Check sheet for the modelled part. Datum: model origin and axes. Units: mm. Face numbers are marked on the shaded views. Give positions to 0.01 mm unless a question says otherwise; leave off trailing zeros. Order: outer loops, then holes, each group sorted by start corner. A loop starts at its lowest first (then second) coordinate and runs counter-clockwise, first axis right, second up.
Item 1: Gauge pin test, flat ends, axial feed: P1, Ø5, axis at y = -15.5, z = 6.5, coming from the +X side; P2, Ø10, axis at x = 28.5, y = -17, coming from the +Z side; P3, Ø3, axis at y = -9.5, z = -18.5, coming from the +X side; P4, Ø6, axis at y = -6, z = -3, coming from the -X side. Record the tip position at first contact, or that the pin passes through.
Item 2: Release check for a two-part mould opening along X. For the marked faces 1 and 2 record: released by +X, released by -X, zero draft, split by the parting line, or undercut.
Item 3: Sectioned sample at A-A on z = -19. Record the boundary of the cut face in (x, y), and give its area (3 significant figures).
Item 4: Material ranges on line 1 along X through (y, z) = (-4, -26.5); line 2 along X through (y, z) = (-16.5, 43); line 3 along Z through (x, y) = (36, -18), recorded low to high.
Item 5: Sectioned sample at C-C on y = -18.25. Record the boundary of the cut face in (x, z), and give its area (3 significant figures).
Item 6: Sectioned sample at B-B on x = -20.5. Record the boundary of the cut face in (y, z), and give its area (3 significant figures).
Item 7: Sectioned sample at D-D on z = 0. Record the boundary of the cut face in (x, y), and give its area (3 significant figures).
from build123d import *

# Parameters (mm, degrees)
SKETCH002_R     = 57.5
PAD002_DEPTH    = 20
SKETCH003_R     = 55
POCKET_DEPTH    = 25
SKETCH004_W     = 65.896674
SKETCH004_H     = 4
POCKET001_DEPTH = 21


with BuildPart() as part:
    # Sketch002 → Pad002 (new body)
    with BuildSketch(Plane.XZ):
        Circle(SKETCH002_R)
    extrude(amount=PAD002_DEPTH)

    # Sketch003 (on Face3 of Pad002) → Pocket (cut)
    with BuildSketch(Plane.XZ.offset(20)):
        with Locations((0.237796, -0.12528)):
            Circle(SKETCH003_R)
    extrude(amount=-POCKET_DEPTH, mode=Mode.SUBTRACT)

    # Sketch004 (on Face3 of Pocket) → Pocket001 (cut)
    with BuildSketch(Plane.XZ.offset(20)):
        with Locations((32.948337, 0)):
            Rectangle(SKETCH004_W, SKETCH004_H)
    extrude(amount=-POCKET001_DEPTH, mode=Mode.SUBTRACT)


with BuildPart() as part_1:
    # Body001 placement: moved
    add(part.part.moved(Location((0, -2, 0))))


solid = part_1.part
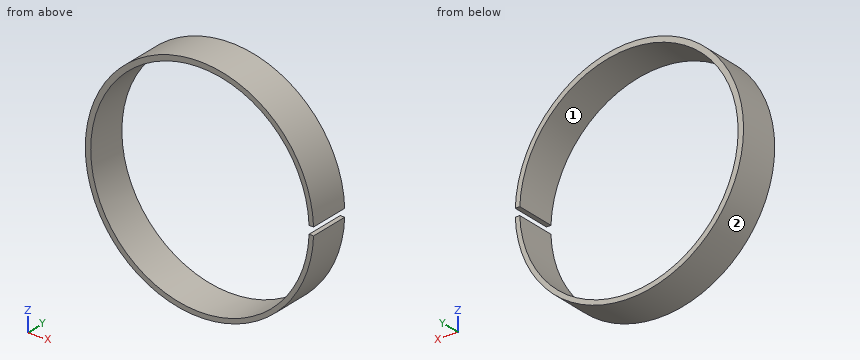
Report:
1. P1: stops at x = 57.36
1. P2: stops at z = 52.48
1. P3: stops at x = 54.93
1. P4: stops at x = -57.5
2. face 1: undercut
2. face 2: split by the parting line
3. outline: (-54.27, -22) - (-51.42, -22) - (-51.42, -2) - (-54.27, -2) - close; (51.9, -22) - (54.27, -22) - (54.27, -2) - (51.9, -2) - close
3. area: 104 mm2
4. line 1: x = -51.03 to -48.03, 48.5 to 51.03
4. line 2: x = -38.17 to -33.9, 34.37 to 38.17
4. line 3: z = -44.84 to -41.91, 41.66 to 44.84
5. outline: (55.2, 2) - (57.47, 2) arc R57.5 ccw (long way) to (57.47, -2) - (55.21, -2) arc R55 cw (long way) to start
5. area: 875 mm2
6. outline: (-22, -53.72) - (-2, -53.72) - (-2, -51.07) - (-22, -51.07) - close; (-22, 50.82) - (-2, 50.82) - (-2, 53.72) - (-22, 53.72) - close
6. area: 111 mm2
7. outline: (-57.5, -22) - (-54.76, -22) - (-54.76, -2) - (-57.5, -2) - close
7. area: 54.8 mm2
